Here's the drawing with two shaded views (mm, measured from the low corner). I have some questions. A direction names the side the tool comes from. Give positions to 0.01 mm unless a question says otherwise; leave off trailing zeros. Write each loop counter-clockwise with the first axis right and the second up, starting at its lowest first coordinate (ties: lowest second). Pieces come first, ordered by that corner, then holes.
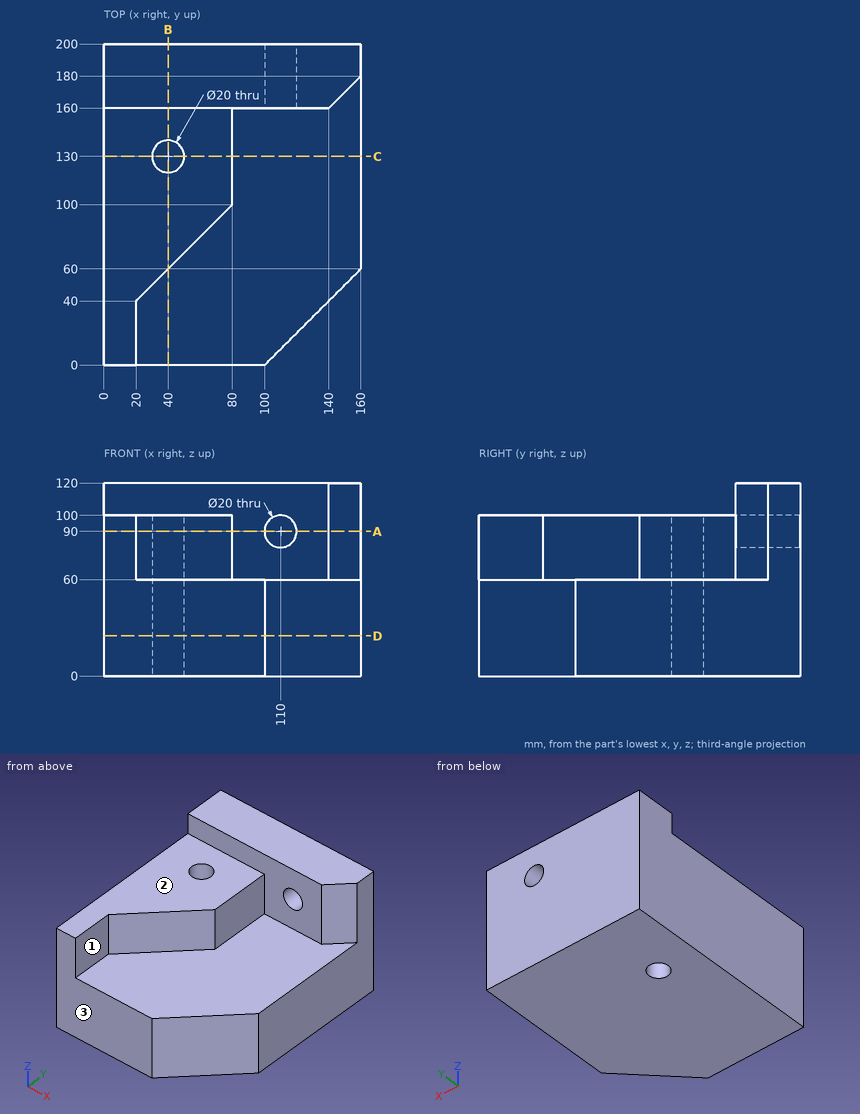
(1) Imagine slicing it at C-C, the plane y = 130. Write out the boundary of the cut face in (x, z).
Returned:
outline: (0, 0) - (30, 0) - (30, 100) - (0, 100) - close; (50, 0) - (160, 0) - (160, 60) - (80, 60) - (80, 100) - (50, 100) - close
(2) Imagine slicing it at A-A, the plane z = 90. Write out the boundary of the cut face in (x, y).
Returned:
outline: (0, 0) - (20, 0) - (20, 40) - (80, 100) - (80, 160) - (100, 160) - (100, 200) - (0, 200) - close; (120, 160) - (140, 160) - (160, 180) - (160, 200) - (120, 200) - close; hole circle Ø20 at (40, 130)
(3) Imagine slicing it at D-D, the plane z = 25. Write out the boundary of the cut face in (x, y).
Returned:
outline: (0, 0) - (100, 0) - (160, 60) - (160, 200) - (0, 200) - close; hole circle Ø20 at (40, 130)
(4) Will these pins go through, and if not, where does the flat tip stop? P1, Ø3, axis at x = 128.5, z = 52.5, coming from the -Y side; P2, Ø6, axis at y = 30, z = 62, coming from the +X side; P3, Ø1, axis at y = 24.5, z = 72, coming from the +X side.
Returned:
P1: stops at y = 27
P2: stops at x = 132.24
P3: stops at x = 20
(5) For the marked faces 1, 2 and 3, which set-ups out of +Z, -Z, +X, -X, +Y, -Y let a thin tool reach every point of the face, with its end or its side?
Returned:
face 1: +Z, +X, -Y
face 2: +Z, +X, -X, -Y
face 3: +Z, -Z, +X, -X, -Y
(6) If I drill on L1, parallel to Y at x = 41, z = 56; L2, parallel to Y at x = 40, z = 37; L3, parallel to Z at x = 110, y = 189, over which ranges is the centre line in solid material (lowest first)?
Returned:
L1: y = 0 to 120.05, 139.95 to 200
L2: y = 0 to 120, 140 to 200
L3: z = 0 to 80, 100 to 120
(7) Imagine slicing it at B-B, the plane x = 40. Write out the boundary of the cut face in (y, z), plus the area to 3 significant figures.
Returned:
outline: (0, 0) - (120, 0) - (120, 100) - (60, 100) - (60, 60) - (0, 60) - close; (140, 0) - (200, 0) - (200, 120) - (160, 120) - (160, 100) - (140, 100) - close
area: 16,400 mm2
